The model under review builds one solid part; all positions refer to its coordinate system, in mm. Face numbers are marked on the shaded views. A direction names the side the tool comes from. Give positions to 0.01 mm unless a question says otherwise; leave off trailing zeros. Order: outer loops, then holes, each group sorted by start corner. A loop starts at its lowest first (then second) coordinate and runs counter-clockwise, first axis right, second up. Notation, with made-up numbers: (44, 46) - (51, 46) arc R19 ccw to (51, 67) - close; hole circle Ø3 at (83, 41). An arc over 180 degrees is marked (long way). Put each result on its own line as item: value.
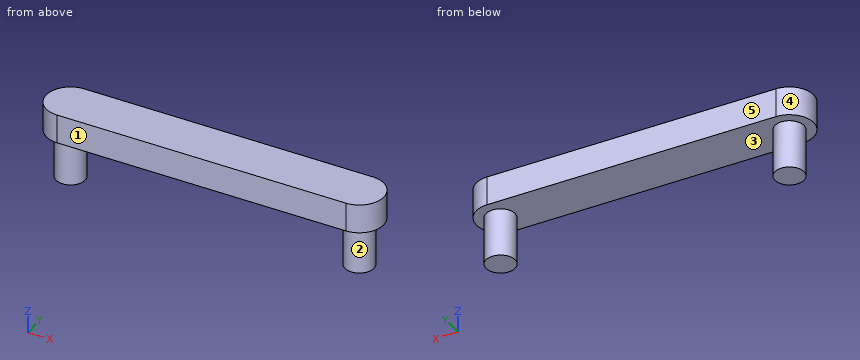
```python
from build123d import *

# Parameters (mm, degrees)
BOSS_EXTRUDE1_DEPTH = 3
SKETCH3_R           = 1.5
BOSS_EXTRUDE2_DEPTH = 5


with BuildPart() as part:
    # Sketch1 → Boss-Extrude1 (new body)
    with BuildSketch(Plane.XY):
        with BuildLine():
            Line((-15, -2.5), (15, -2.5))
            ThreePointArc((15, -2.5), (17.5, 0), (15, 2.5))
            Line((15, 2.5), (-15, 2.5))
            ThreePointArc((-15, 2.5), (-17.5, 0), (-15, -2.5))
        make_face()
    extrude(amount=BOSS_EXTRUDE1_DEPTH)

    # Sketch3 → Boss-Extrude2 (add)
    with BuildSketch(Plane.XY):
        with Locations((-15, 0)):
            Circle(SKETCH3_R)
        with Locations((15, 0)):
            Circle(SKETCH3_R)
    extrude(amount=-BOSS_EXTRUDE2_DEPTH)


solid = part.part
```
(1) Clearance check with flat-ended pins moving along their axes: pin 1 Ø4 at (x, z) = (7.5, -2.5) entering from -Y; pin 2 Ø1 at (y, z) = (1, 2) entering from +X; pin 3 Ø1.5 at (y, z) = (-1, 2) entering from -X; pin 4 Ø3 at (x, y) = (-9, 1) entering from -Z. State where each tip first meets the part, or that it passes through.
The answers:
pin 1: through
pin 2: x = 17.45
pin 3: x = -17.49
pin 4: z = 0
(2) Wall thickness on L1, parallel to Z at x = 6.5, y = 0.2; L2, parallel to X at y = -0.7, z = -2.5; L3, parallel to X at y = 0.1, z = 1.25: over which ranges is each line inside the solid? List them lowest first.
The answers:
L1: 0 to 3
L2: -16.33 to -13.67, 13.67 to 16.33
L3: -17.5 to 17.5
(3) The part is to be moulded in two halves that separate along X. For the marked faces 3, 4 and 5, say which applies: pulls with the +X half, pulls with the -X half, needs draft (parallel to the pull), parting line crosses it, or undercut.
The answers:
face 3: undercut
face 4: pulls with the -X half
face 5: needs draft
(4) Take a section at A-A, the plane y = 0. Write out the cut boundary in (x, z), then the cut area to 3 significant figures.
The answers:
outline: (-17.5, 0) - (-16.5, 0) - (-16.5, -5) - (-13.5, -5) - (-13.5, 0) - (13.5, 0) - (13.5, -5) - (16.5, -5) - (16.5, 0) - (17.5, 0) - (17.5, 3) - (-17.5, 3) - close
area: 135 mm^2
(5) For the marked faces 1 and 2, list the 3-axis set-ups (+Z, -Z, +X, -X, +Y, -Y) from which the entire face can be reached by the end or side of a thin tool; tool diameter is ignored.
The answers:
face 1: +Z, -Z, +X, -X, -Y
face 2: -Z
(6) Take a section at D-D, the plane z = 1.5. Write out the cut boundary in (x, y), then the cut area to 3 significant figures.
The answers:
outline: (-15, -2.5) - (15, -2.5) arc R2.5 ccw to (15, 2.5) - (-15, 2.5) arc R2.5 ccw to start
area: 170 mm^2
(7) Take a section at C-C, the plane x = 8. Write out the cut boundary in (y, z), then the cut area to 3 significant figures.
The answers:
outline: (-2.5, 0) - (2.5, 0) - (2.5, 3) - (-2.5, 3) - close
area: 15.0 mm^2
(8) Take a section at B-B, the plane z = -2.5. Write out the cut boundary in (x, y).
The answers:
outline: circle Ø3 at (-15, 0); circle Ø3 at (15, 0)
